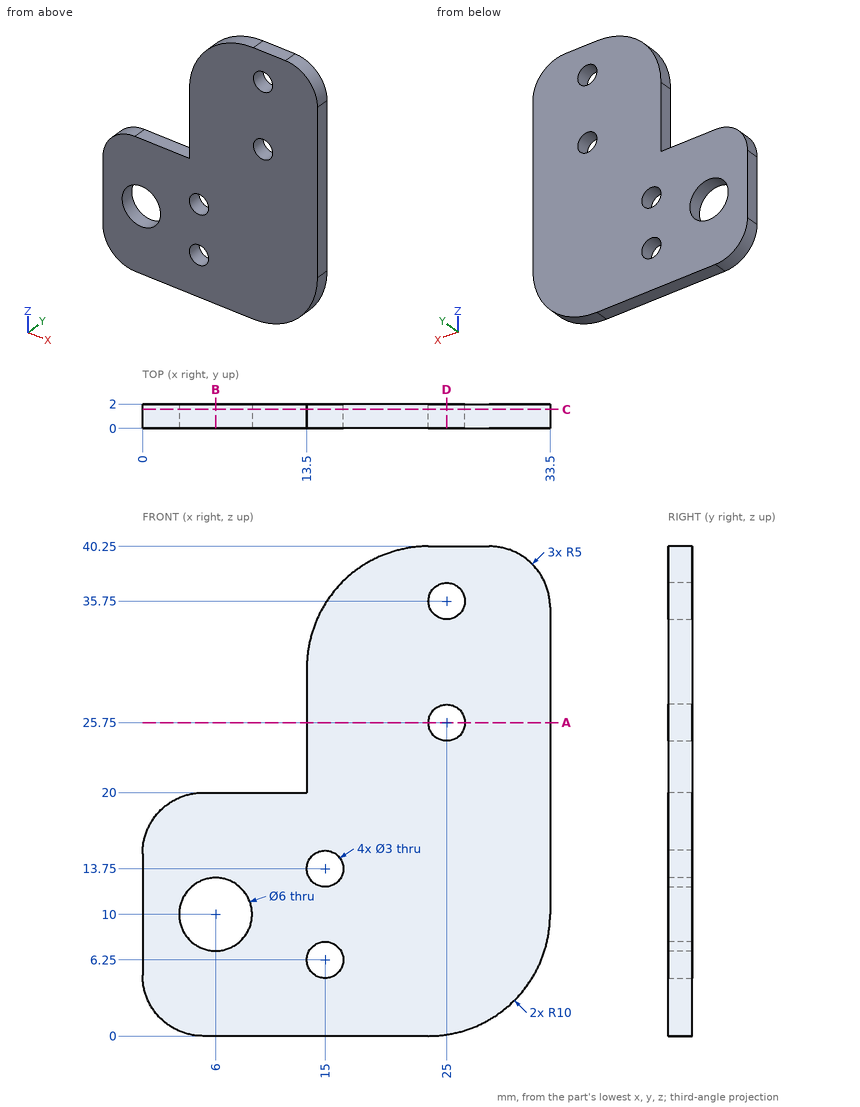
Geometry: see drawing. Coordinates: mm, zero at the bounding-box minimum. Coordinates: 2 decimals unless noted, no trailing zeros. Write each loop counter-clockwise with the first axis right and the second up, starting at its lowest first coordinate (ties: lowest second). Pieces come first, ordered by that corner, then holes. Notation, with made-up numbers: M 12.5,79 L 18.5,79 A21 cw 18.5,117 Z; hole C -10,85 d2. An arc over 180 degrees is marked long. Use CSV: the item, a comma, the result in double quotes. Start each with the question number.
1. Cut plane C-C on y = 1.55. Return the cut outline in (x, z).
2. Cut plane B-B on x = 6. Return the cut outline in (y, z), plus the area to 3 significant figures.
3. Ray query, probe 1 along X at (y, z) = (0.7, 13.75); probe 2 along X at (y, z) = (0.4, 36); probe 3 along X at (y, z) = (1.1, 29). Return the intervals inside material, ascending.
4. Cut plane A-A on z = 25.75. Return the cut outline in (x, y), plus the area to 3 significant figures.
5. First-contact query: P1, Ø1, axis at y = 0.5, z = 4, coming from the +X side; P2, Ø1, axis at y = 1.5, z = 22.5, coming from the -X side. Flat tips, straight axial feed; report the tip coordinate or a pass-through.
6. Cut plane D-D on x = 25. Return the cut outline in (y, z), plus the area to 3 significant figures.
Entries:
1,outline,"M 0,5 A5 ccw 5,0 L 23.5,0 A10 ccw 33.5,10 L 33.5,35.25 A5 ccw 28.5,40.25 L 23.5,40.25 A10 ccw 13.5,30.25 L 13.5,20 L 5,20 A5 ccw 0,15 Z; hole C 6,10 d6; hole C 15,6.25 d3; hole C 15,13.75 d3; hole C 25,25.75 d3; hole C 25,35.75 d3"
2,outline,"M 0,0 L 2,0 L 2,7 L 0,7 Z; M 0,13 L 2,13 L 2,20 L 0,20 Z"
2,area,"28.0 mm²"
3,probe 1,"0 to 13.5, 16.5 to 33.5"
3,probe 2,"15.32 to 23.52, 26.48 to 33.44"
3,probe 3,"13.5 to 33.5"
4,outline,"M 13.5,0 L 23.5,0 L 23.5,2 L 13.5,2 Z; M 26.5,0 L 33.5,0 L 33.5,2 L 26.5,2 Z"
4,area,"34.0 mm²"
5,P1,"x = 31.85"
5,P2,"x = 13.5"
6,outline,"M 0,0.11 L 2,0.11 L 2,24.25 L 0,24.25 Z; M 0,27.25 L 2,27.25 L 2,34.25 L 0,34.25 Z; M 0,37.25 L 2,37.25 L 2,40.25 L 0,40.25 Z"
6,area,"68.3 mm²"
